Design review of the part shown in the three views and the two pictorial views. Dimensions are in mm from the part's minimum x, y and z. A direction names the side the tool comes from. Give positions to 0.01 mm unless a question says otherwise; leave off trailing zeros. Loops run counter-clockwise (first coordinate to the right, second up) from the corner with the lowest first, then second, coordinate; pieces in that order, holes last. Notation, with made-up numbers: (70.25, -13.5) -> (120.25, -13.5) arc R31 cw to (120.25, 21.5) -> close; hole circle Ø4 at (27, 63.25). An arc over 180 degrees is marked (long way). Answer as CSV lines item,"result". Start each with the question number.
Item 1: Clearance check with flat-ended pins moving along their axes: P1, Ø1, axis at y = 50, z = 4.5, coming from the +X side; P2, Ø3, axis at x = 27.5, z = 15.5, coming from the +Y side; P3, Ø4, axis at y = 39.5, z = 16, coming from the +X side. State where each tip first meets the part, or that it passes through.
Item 2: Add section C-C on y = 50. State the section outline as (x, z) points, plus the area to 3 significant figures.
Item 3: For L1, parallel to Y at x = 30, z = 8; L2, parallel to Z at x = 56.5, y = 28.5; L3, parallel to Y at x = 27.5, z = 6.25 (1 decimal), list the stretches that pass through material, from the lowest coordinate up. Write a range as from..to.
Item 4: Machinability: for the marked faces 4, 5, 6, 7 and 8, which of the approach directions +Z, -Z, +X, -X, +Y, -Y give a long, thin tool a straight path to every point of the face, cutting with its end or side? Answer none if there is none.
Item 5: Add section A-A on z = 12.25. State the section outline as (x, y) points.
Item 6: Add section B-B on x = 30. State the section outline as (y, z) points, plus the area to 3 significant figures.
Item 7: Add section D-D on y = 43. State the section outline as (x, z) points (1 decimal), plus the area to 3 significant figures.
Item 8: The part is to be moulded in two halves that separate along Y. For the marked faces 1, 2 and 3, say which applies: +Y half, -Y half, draft (parallel to the pull), parting line (faces both ways), or undercut.
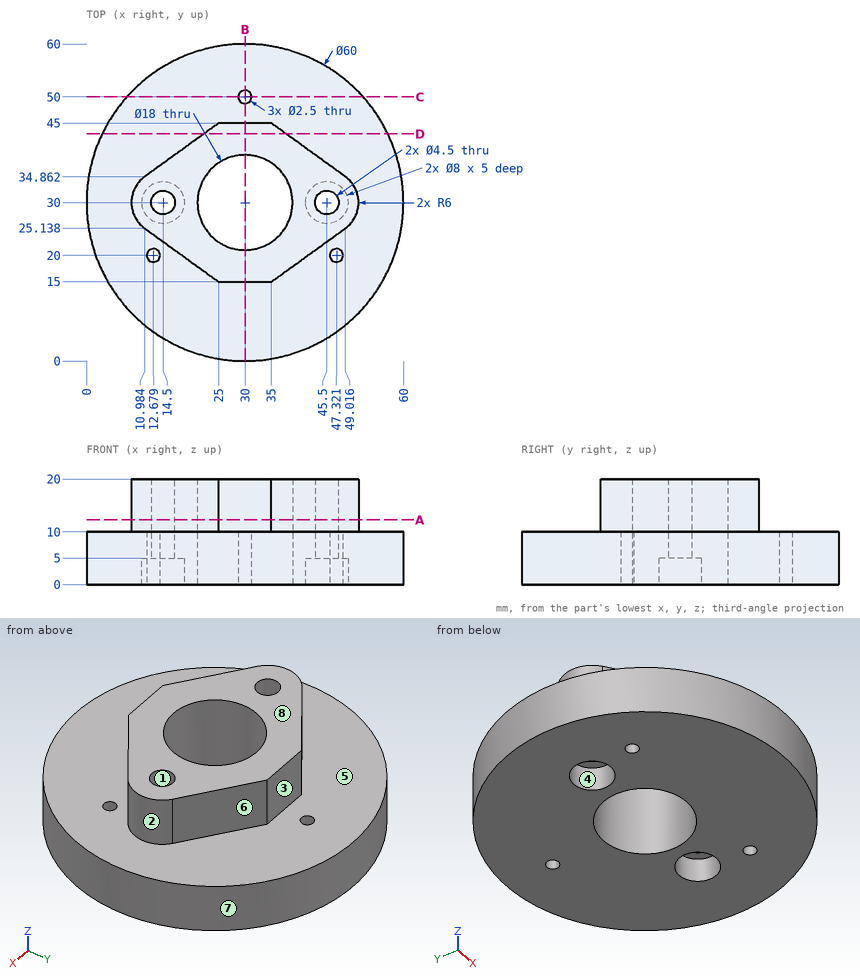
Computed values:
1,P1,"x = 52.8"
1,P2,"y = 45"
1,P3,"x = 45.37"
2,outline,"(7.64, 0) -> (28.75, 0) -> (28.75, 10) -> (7.64, 10) -> close; (31.25, 0) -> (52.36, 0) -> (52.36, 10) -> (31.25, 10) -> close"
2,area,"422 mm²"
3,L1,"0..21, 39..48.75, 51.25..60"
3,L2,"0..10"
3,L3,"0.1..21.4, 38.6..59.9"
4,face 4,"-Z"
4,face 5,"+Z"
4,face 6,"+Z, +X, +Y"
4,face 7,"+Z, -Z"
4,face 8,"+Z, +X, -X, +Y, -Y"
5,outline,"(10.98, 25.14) -> (25, 15) -> (35, 15) -> (49.02, 25.14) arc R6 ccw to (49.02, 34.86) -> (35, 45) -> (25, 45) -> (10.98, 34.86) arc R6 ccw to start; hole circle Ø4.5 at (14.5, 30); hole circle Ø18 at (30, 30); hole circle Ø4.5 at (45.5, 30)"
6,outline,"(0, 0) -> (21, 0) -> (21, 20) -> (15, 20) -> (15, 10) -> (0, 10) -> close; (39, 0) -> (48.75, 0) -> (48.75, 10) -> (45, 10) -> (45, 20) -> (39, 20) -> close; (51.25, 0) -> (60, 0) -> (60, 10) -> (51.25, 10) -> close"
6,area,"515 mm²"
7,outline,"(3, 0) -> (57, 0) -> (57, 10) -> (37.8, 10) -> (37.8, 20) -> (22.2, 20) -> (22.2, 10) -> (3, 10) -> close"
7,area,"696 mm²"
8,face 1,"undercut"
8,face 2,"parting line"
8,face 3,"+Y half"
